Model file for the job. Use its own axes, mm. A direction names the side the tool comes from. Round coordinates to 2 decimals unless told otherwise and drop trailing zeros. Order: outer loops, then holes, each group sorted by start corner. A loop starts at its lowest first (then second) coordinate and runs counter-clockwise, first axis right, second up. Notation, with made-up numbers: (74.5, 82) - (109.5, 82) arc R25 cw to (109.5, 117) - close; hole circle Ø3 at (-1, 27.5). An arc over 180 degrees is marked (long way). Answer as CSV lines item,"result". Start each with the question number.
1. Wall check: line 1 along Z through (x, y) = (5.5, 1); line 2 along X through (y, z) = (3.5, 1.5). Give the ranges that are in metal, low to high. Write a range as [from, to].
2. Band-saw the part on C-C on x = 5.5. State how many separate pieces and enclosed holes the cut face has, then the cut area to 3 significant figures.
3. Band-saw the part on A-A on x = 0. List the corners of the cut face in (y, z).
4. Band-saw the part on B-B on z = 0. List the corners of the cut face in (x, y).
5. Pin check, flat tips, straight feed: pin 1 Ø2.5 at (x, y) = (4.5, 2) entering from +Z; pin 2 Ø1.8 at (y, z) = (-1, 4.5) entering from +X; pin 3 Ø0.6 at (y, z) = (-0.5, -1.5) entering from +X. Stop position of each tip, or through.
6. 3-axis set-ups, long thin cutter, end or side, ignore diameter. For faces 4 (the face through (4.71, 0.05, -1.97)), 5 (the face through (-1.97, 0.05, -4.71)), 6 (the face through (-1, 0.1, 1.5)), 7 (the face through (0.65, 0, 5)): which of +Z, -Z, +X, -X, +Y, -Y reach the whole face in a straight line?
7. Pull direction X, two halves, no side cores. Call faces 1 (the face through (1, 0.1, -1.5)), 2 (the face through (3, -3.6, 5.1)), 3 (the face through (5, 0, -0.65)): released by +X, released by -X, zero draft, split by the parting line, or undercut.
```python
from build123d import *

# Parameters (mm, degrees)
SKETCH1_R           = 4
BOSS_EXTRUDE1_DEPTH = 3.9
BOSS_EXTRUDE2_DEPTH = 7.8
CIRPATTERN1_COUNT   = 12
SKETCH7_W           = 2
SKETCH7_H           = 2
CUT_EXTRUDE2_DEPTH  = 8.8
FILLET4_R           = 1
FILLET5_R           = 1
FILLET6_R           = 1
FILLET7_R           = 1
FILLET8_R           = 1
FILLET9_R           = 1
FILLET10_R          = 1
FILLET11_R          = 1
FILLET12_R          = 1
FILLET13_R          = 1
FILLET14_R          = 1
FILLET15_R          = 1
FILLET16_R          = 1
FILLET17_R          = 1
FILLET18_R          = 1
FILLET19_R          = 1
FILLET20_R          = 1
FILLET21_R          = 1
FILLET22_R          = 1
FILLET23_R          = 1
FILLET24_R          = 1
FILLET25_R          = 1
FILLET26_R          = 1
FILLET27_R          = 1


with BuildPart() as part:
    # Sketch1 → Boss-Extrude1 (new body, symmetric)
    with BuildSketch(Plane(origin=(0, 0, 0), x_dir=(1, 0, 0), z_dir=(0, 1, 0))):
        Circle(SKETCH1_R)
    extrude(amount=BOSS_EXTRUDE1_DEPTH, both=True)

    # Sketch5 → Boss-Extrude2 (add)
    with BuildSketch(Plane(origin=(0, 3.9, 0), x_dir=(1, 0, 0), z_dir=(0, 1, 0))):
        with BuildLine():
            ThreePointArc((-0.65, 3.946834174), (-0.326085344, 3.986686387), (0, 4))
            Line((0, 4), (0, 6.2))
            Line((0, 6.2), (-0.65, 6.2))
            Line((-0.65, 6.2), (-0.65, 3.946834174))
        make_face()
        with BuildLine():
            Line((0, 6.2), (0, 4))
            ThreePointArc((0, 4), (0.326085344, 3.986686387), (0.65, 3.946834174))
            Line((0.65, 3.946834174), (0.65, 6.2))
            Line((0.65, 6.2), (0, 6.2))
        make_face()
    boss_extrude2 = extrude(amount=-BOSS_EXTRUDE2_DEPTH)

    # CirPattern1: Boss-Extrude2 ×12 about axis
    cirpattern1_axis = Axis((0, 0, 0), (0, 1, 0))
    for i in range(1, CIRPATTERN1_COUNT):
        add(boss_extrude2.rotate(cirpattern1_axis, i * 360 / CIRPATTERN1_COUNT))

    # Sketch7 → Cut-Extrude2 (cut, through all)
    with BuildSketch(Plane(origin=(0, 3.9, 0), x_dir=(1, 0, 0), z_dir=(0, 1, 0))):
        with BuildLine():
            Line((1, 1), (1, 2.1))
            ThreePointArc((1, 2.1), (0, 3.1), (-1, 2.1))
            Line((-1, 2.1), (-1, 1))
            Line((-1, 1), (1, 1))
        make_face()
        Rectangle(SKETCH7_W, SKETCH7_H)
        with BuildLine():
            Line((1.9, 1), (1, 1))
            Line((1, 1), (1, -1))
            Line((1, -1), (1.9, -1))
            ThreePointArc((1.9, -1), (2.9, 0), (1.9, 1))
        make_face()
        with BuildLine():
            Line((1, -2.1), (1, -1))
            Line((1, -1), (-1, -1))
            Line((-1, -1), (-1, -2.1))
            ThreePointArc((-1, -2.1), (0, -3.1), (1, -2.1))
        make_face()
        with BuildLine():
            Line((-1, -1), (-1, 1))
            Line((-1, 1), (-2.1, 1))
            ThreePointArc((-2.1, 1), (-3.1, 0), (-2.1, -1))
            Line((-2.1, -1), (-1, -1))
        make_face()
    extrude(amount=-CUT_EXTRUDE2_DEPTH, mode=Mode.SUBTRACT)

    # Fillet4
    fillet4_edges = [part.edges().sort_by_distance(p)[0] for p in [
        (3.1, 3.9, -5.369357503),
    ]]
    fillet(fillet4_edges, radius=FILLET4_R)

    # Fillet5
    fillet5_edges = [part.edges().sort_by_distance(p)[0] for p in [
        (5.369357503, 3.9, 3.1),
    ]]
    fillet(fillet5_edges, radius=FILLET5_R)

    # Fillet6
    fillet6_edges = [part.edges().sort_by_distance(p)[0] for p in [
        (6.2, 3.9, 0),
    ]]
    fillet(fillet6_edges, radius=FILLET6_R)

    # Fillet7
    fillet7_edges = [part.edges().sort_by_distance(p)[0] for p in [
        (5.369357503, -3.9, -3.1),
    ]]
    fillet(fillet7_edges, radius=FILLET7_R)

    # Fillet8
    fillet8_edges = [part.edges().sort_by_distance(p)[0] for p in [
        (3.1, -3.9, 5.369357503),
    ]]
    fillet(fillet8_edges, radius=FILLET8_R)

    # Fillet9
    fillet9_edges = [part.edges().sort_by_distance(p)[0] for p in [
        (3.1, 3.9, 5.369357503),
    ]]
    fillet(fillet9_edges, radius=FILLET9_R)

    # Fillet10
    fillet10_edges = [part.edges().sort_by_distance(p)[0] for p in [
        (0, 3.9, 6.2),
    ]]
    fillet(fillet10_edges, radius=FILLET10_R)

    # Fillet11
    fillet11_edges = [part.edges().sort_by_distance(p)[0] for p in [
        (-3.1, 3.9, 5.369357503),
    ]]
    fillet(fillet11_edges, radius=FILLET11_R)

    # Fillet12
    fillet12_edges = [part.edges().sort_by_distance(p)[0] for p in [
        (-5.369357503, 3.9, 3.1),
    ]]
    fillet(fillet12_edges, radius=FILLET12_R)

    # Fillet13
    fillet13_edges = [part.edges().sort_by_distance(p)[0] for p in [
        (-6.2, 3.9, 0),
    ]]
    fillet(fillet13_edges, radius=FILLET13_R)

    # Fillet14
    fillet14_edges = [part.edges().sort_by_distance(p)[0] for p in [
        (-3.1, 3.9, -5.369357503),
    ]]
    fillet(fillet14_edges, radius=FILLET14_R)

    # Fillet15
    fillet15_edges = [part.edges().sort_by_distance(p)[0] for p in [
        (-5.369357503, 3.9, -3.1),
    ]]
    fillet(fillet15_edges, radius=FILLET15_R)

    # Fillet16
    fillet16_edges = [part.edges().sort_by_distance(p)[0] for p in [
        (0, 3.9, -6.2),
    ]]
    fillet(fillet16_edges, radius=FILLET16_R)

    # Fillet17
    fillet17_edges = [part.edges().sort_by_distance(p)[0] for p in [
        (5.369357503, 3.9, -3.1),
    ]]
    fillet(fillet17_edges, radius=FILLET17_R)

    # Fillet18
    fillet18_edges = [part.edges().sort_by_distance(p)[0] for p in [
        (-6.2, -3.9, 0),
    ]]
    fillet(fillet18_edges, radius=FILLET18_R)

    # Fillet19
    fillet19_edges = [part.edges().sort_by_distance(p)[0] for p in [
        (-5.369357503, -3.9, 3.1),
    ]]
    fillet(fillet19_edges, radius=FILLET19_R)

    # Fillet20
    fillet20_edges = [part.edges().sort_by_distance(p)[0] for p in [
        (-3.1, -3.9, 5.369357503),
    ]]
    fillet(fillet20_edges, radius=FILLET20_R)

    # Fillet21
    fillet21_edges = [part.edges().sort_by_distance(p)[0] for p in [
        (0, -3.9, 6.2),
    ]]
    fillet(fillet21_edges, radius=FILLET21_R)

    # Fillet22
    fillet22_edges = [part.edges().sort_by_distance(p)[0] for p in [
        (5.369357503, -3.9, 3.1),
    ]]
    fillet(fillet22_edges, radius=FILLET22_R)

    # Fillet23
    fillet23_edges = [part.edges().sort_by_distance(p)[0] for p in [
        (6.2, -3.9, 0),
    ]]
    fillet(fillet23_edges, radius=FILLET23_R)

    # Fillet24
    fillet24_edges = [part.edges().sort_by_distance(p)[0] for p in [
        (0, -3.9, -6.2),
    ]]
    fillet(fillet24_edges, radius=FILLET24_R)

    # Fillet25
    fillet25_edges = [part.edges().sort_by_distance(p)[0] for p in [
        (-3.1, -3.9, -5.369357503),
    ]]
    fillet(fillet25_edges, radius=FILLET25_R)

    # Fillet26
    fillet26_edges = [part.edges().sort_by_distance(p)[0] for p in [
        (3.1, -3.9, -5.369357503),
    ]]
    fillet(fillet26_edges, radius=FILLET26_R)

    # Fillet27
    fillet27_edges = [part.edges().sort_by_distance(p)[0] for p in [
        (-5.369357503, -3.9, -3.1),
    ]]
    fillet(fillet27_edges, radius=FILLET27_R)


solid = part.part
```
Reply:
1,line 1,"z = [-2.87, -2.42], [-0.65, 0.65], [2.42, 2.87]"
1,line 2,"x = [-3.9, -1], [1, 3.9]"
2,separate pieces,"3"
2,enclosed holes,"0"
2,area,"16.0 mm2"
3,outline,"(-3.9, -5.2) arc R1 ccw to (-2.9, -6.2) - (2.9, -6.2) arc R1 ccw to (3.9, -5.2) - (3.9, -3.1) - (-3.9, -3.1) - close; (-3.9, 3.1) - (3.9, 3.1) - (3.9, 5.2) arc R1 ccw to (2.9, 6.2) - (-2.9, 6.2) arc R1 ccw to (-3.9, 5.2) - close"
4,outline,"(-6.2, -2.9) arc R1 ccw to (-5.2, -3.9) - (-3.1, -3.9) - (-3.1, 3.9) - (-5.2, 3.9) arc R1 ccw to (-6.2, 2.9) - close; (2.9, -3.9) - (5.2, -3.9) arc R1 ccw to (6.2, -2.9) - (6.2, 2.9) arc R1 ccw to (5.2, 3.9) - (2.9, 3.9) - close"
5,pin 1,"stops at z = 5.28"
5,pin 2,"stops at x = 5.08"
5,pin 3,"stops at x = 4.42"
6,face 4,"+X, +Y, -Y"
6,face 5,"-Z, +Y, -Y"
6,face 6,"+Y, -Y"
6,face 7,"+Z, +Y, -Y"
7,face 1,"undercut"
7,face 2,"released by +X"
7,face 3,"zero draft"
